Work out the finished part from the listing and answer in its coordinate system (mm). Face numbers are marked on the shaded views. A direction names the side the tool comes from. Round coordinates to 2 decimals unless told otherwise and drop trailing zeros. Loops run counter-clockwise (first coordinate to the right, second up) from the corner with the lowest first, then second, coordinate; pieces in that order, holes last. Notation, with made-up numbers: (28, 66.5) - (68, 66.5) arc R22 cw to (68, 93.5) - close; hole circle Ø11 at (43.5, 86). An arc over 180 degrees is marked (long way). Answer as CSV lines item,"result". Start each with the question number.
Q1. For the marked faces 5, 6 and 7, determine the directions among +Z, -Z, +X, -X, +Y, -Y from which every point of the face is accessible in a straight line to the end or side of a thin tool.
Q2. Section B-B on z = 9 is taken. Write down the section's boundary in (x, y).
Q3. Section C-C on x = 8.6 is taken. Write down the section's boundary in (y, z), then the cut area to 3 significant figures.
Q4. Each of these flat-tipped pins is pushed along its axis until it touches: pin 1 Ø8 at (x, z) = (-7, 4.5) entering from +Y; pin 2 Ø4.5 at (y, z) = (8.11, 9) entering from -X; pin 3 Ø2 at (x, z) = (1.5, 2) entering from +Y. Where does it stop, or does it pass through?
Q5. The mould has two halves that part along Y. Classify the marked faces 1, 2, 3 and 4: +Y half, -Y half, draft (parallel to the pull), parting line (faces both ways), or undercut.
Q6. Section A-A on y = 0 is taken. Write down the section's boundary in (x, z), then the cut area to 3 significant figures.
Q7. Straight lines are drawn through the part: L1, parallel to X at y = 0, z = 7.5; L2, parallel to X at y = 5.5, z = 6.75; L3, parallel to X at y = 1, z = 3.25. For each, find the intervals that lie inside material, in ascending order. Write a range as [from, to].
Q8. Section D-D on z = 4.75 is taken. Write down the section's boundary in (x, y).
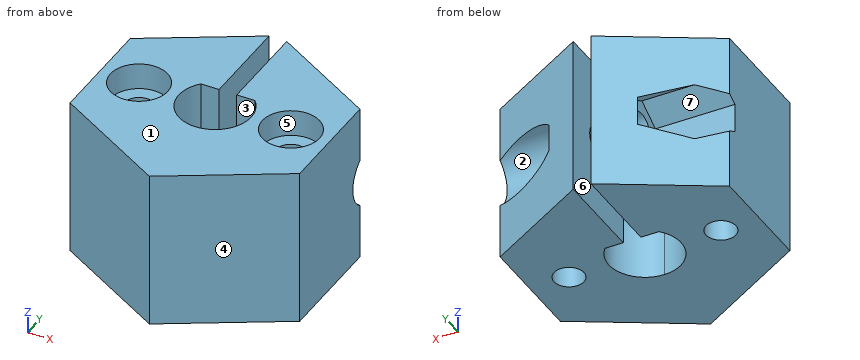
```python
from build123d import *

# Parameters (mm, degrees)
BOSS_EXTRUDE1_DEPTH            = 18
SKETCH41_R                     = 1.7
CUT_EXTRUDE7_DEPTH             = 18
CBORE_FOR_M3_SHCS1_D           = 3.4
CBORE_FOR_M3_SHCS1_CBORE_D     = 6.5
CBORE_FOR_M3_SHCS1_CBORE_DEPTH = 3
CBORE_FOR_M3_SHCS2_D           = 3.4
CBORE_FOR_M3_SHCS2_CBORE_D     = 6.5
CBORE_FOR_M3_SHCS2_CBORE_DEPTH = 3
SKETCH52_R                     = 1.7
CUT_EXTRUDE10_DEPTH            = 15
CUT_EXTRUDE10_DEPTH_BACK       = 15
SKETCH58_R                     = 3.25
CUT_EXTRUDE11_DEPTH            = 8
CUT_EXTRUDE12_DEPTH            = 4
CUT_EXTRUDE12_DEPTH_BACK       = 6


with BuildPart() as part:
    # Sketch1 → Boss-Extrude1 (new body)
    with BuildSketch(Plane(origin=(0, 0, 0), x_dir=(0, 1, 0), z_dir=(0, 0, 1))):
        with BuildLine():
            Line((-6.350852961, -13), (6.350852961, -13))
            Line((6.350852961, -13), (13.279056191, -1))
            Line((13.279056191, -1), (2.724986242, -1))
            Line((2.724986242, -1), (2.724986242, -3.063404965))
            ThreePointArc((2.724986242, -3.063404965), (-1.678921738, -3.740484166), (-4.1, 0))
            ThreePointArc((-4.1, 0), (-1.678921738, 3.740484166), (2.724986242, 3.063404965))
            Line((2.724986242, 3.063404965), (2.724986242, 1))
            Line((2.724986242, 1), (13.279056191, 1))
            Line((13.279056191, 1), (6.350852961, 13))
            Line((6.350852961, 13), (-6.350852961, 13))
            Line((-6.350852961, 13), (-13.856406461, 0))
            Line((-13.856406461, 0), (-6.350852961, -13))
        make_face()
    extrude(amount=BOSS_EXTRUDE1_DEPTH)

    # Sketch41 → Cut-Extrude7 (cut)
    with BuildSketch(Plane(origin=(0, 0, 0), x_dir=(0, 1, 0), z_dir=(0, 0, 1))):
        with Locations((0, 8.6)):
            Circle(SKETCH41_R)
        with Locations((0, -8.6)):
            Circle(SKETCH41_R)
    extrude(amount=CUT_EXTRUDE7_DEPTH, mode=Mode.SUBTRACT)

    # CBORE for M3 SHCS1 (through all)
    with Locations(Plane(origin=(-8.6, 0, 18), x_dir=(1, 0, 0), z_dir=(0, 0, 1))):
        with Locations((0, 0)):
            CounterBoreHole(CBORE_FOR_M3_SHCS1_D / 2, CBORE_FOR_M3_SHCS1_CBORE_D / 2, CBORE_FOR_M3_SHCS1_CBORE_DEPTH)

    # CBORE for M3 SHCS2 (through all)
    with Locations(Plane(origin=(8.6, 0, 18), x_dir=(1, 0, 0), z_dir=(0, 0, 1))):
        with Locations((0, 0)):
            CounterBoreHole(CBORE_FOR_M3_SHCS2_D / 2, CBORE_FOR_M3_SHCS2_CBORE_D / 2, CBORE_FOR_M3_SHCS2_CBORE_DEPTH)

    # Sketch52 → Cut-Extrude10 (cut, two sides)
    with BuildSketch(Plane.YZ.offset(-1)) as cut_extrude10_sk:
        with Locations((8.106406461, 9)):
            Circle(SKETCH52_R)
    extrude(amount=CUT_EXTRUDE10_DEPTH, mode=Mode.SUBTRACT)
    extrude(cut_extrude10_sk.sketch, amount=-CUT_EXTRUDE10_DEPTH_BACK, mode=Mode.SUBTRACT)

    # Sketch58 → Cut-Extrude11 (cut)
    with BuildSketch(Plane.YZ.offset(13)):
        with Locations((8.106406461, 9)):
            Circle(SKETCH58_R)
    extrude(amount=-CUT_EXTRUDE11_DEPTH, mode=Mode.SUBTRACT)

    # Sketch60 → Cut-Extrude12 (cut, two sides)
    with BuildSketch(Plane.YZ.offset(-8)) as cut_extrude12_sk:
        Polygon((8.106406461, 5.709103466), (10.956406461, 7.354551733), (10.956406461, 10.645448267), (8.106406461, 12.290896534), (5.256406461, 10.645448267), (5.256406461, 7.354551733), align=None)
    extrude(amount=CUT_EXTRUDE12_DEPTH, mode=Mode.SUBTRACT)
    extrude(cut_extrude12_sk.sketch, amount=-CUT_EXTRUDE12_DEPTH_BACK, mode=Mode.SUBTRACT)


solid = part.part
```
Findings:
1,face 5,"+Z"
1,face 6,"+Z, -Z, +Y"
1,face 7,"-X"
2,outline,"(-13, -6.35) - (0, -13.86) - (13, -6.35) - (13, 4.86) - (5, 4.86) - (5, 6.41) - (1, 6.41) - (1, 2.72) - (3.06, 2.72) arc R4.1 cw (long way) to (-3.06, 2.72) - (-1, 2.72) - (-1, 6.41) - (-4, 6.41) - (-4, 5.26) - (-13, 5.26) - close; (-5.02, 10.96) - (-4, 10.96) - (-4, 9.81) - (-1, 9.81) - (-1, 13.28) - close; (1, 9.81) - (5, 9.81) - (5, 10.97) - (1, 13.28) - close; hole circle Ø3.4 at (-8.6, 0); hole circle Ø3.4 at (8.6, 0)"
3,outline,"(-8.89, 0) - (-1.7, 0) - (-1.7, 15) - (-3.25, 15) - (-3.25, 18) - (-8.89, 18) - close; (1.7, 0) - (8.89, 0) - (8.89, 5.85) arc R3.25 cw (long way) to (8.89, 12.15) - (8.89, 18) - (3.25, 18) - (3.25, 15) - (1.7, 15) - close"
3,area,"228 mm^2"
4,pin 1,"stops at y = 12.12"
4,pin 2,"stops at x = -4"
4,pin 3,"stops at y = 13.28"
5,face 1,"draft"
5,face 2,"undercut"
5,face 3,"undercut"
5,face 4,"-Y half"
6,outline,"(-13, 0) - (-10.3, 0) - (-10.3, 15) - (-11.85, 15) - (-11.85, 18) - (-13, 18) - close; (-6.9, 0) - (-4.1, 0) - (-4.1, 18) - (-5.35, 18) - (-5.35, 15) - (-6.9, 15) - close; (4.1, 0) - (6.9, 0) - (6.9, 15) - (5.35, 15) - (5.35, 18) - (4.1, 18) - close; (10.3, 0) - (13, 0) - (13, 18) - (11.85, 18) - (11.85, 15) - (10.3, 15) - close"
6,area,"179 mm^2"
7,L1,"x = [-13, -10.3], [-6.9, -4.1], [4.1, 6.9], [10.3, 13]"
7,L2,"x = [-13, -1], [1, 13]"
7,L3,"x = [-13, -9.97], [-7.23, -3.98], [3.98, 7.23], [9.97, 13]"
8,outline,"(-13, -6.35) - (0, -13.86) - (13, -6.35) - (13, 6.35) - (1, 13.28) - (1, 2.72) - (3.06, 2.72) arc R4.1 cw (long way) to (-3.06, 2.72) - (-1, 2.72) - (-1, 13.28) - (-13, 6.35) - close; hole circle Ø3.4 at (-8.6, 0); hole circle Ø3.4 at (8.6, 0)"
